Check sheet for the modelled part. Datum: model origin and axes. Units: mm. Face numbers are marked on the shaded views. A direction names the side the tool comes from. Round coordinates to 2 decimals unless told otherwise and drop trailing zeros. Write each loop counter-clockwise with the first axis right and the second up, starting at its lowest first coordinate (ties: lowest second). Pieces come first, ordered by that corner, then holes.
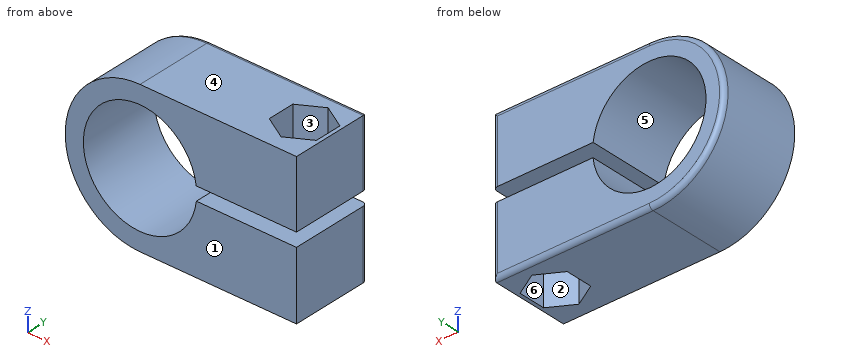
from build123d import *

# Parameters (mm, degrees)
BOSS_EXTRUDE1_DEPTH = 18
FILLET1_R           = 1
CUT_EXTRUDE1_START  = -10
CUT_EXTRUDE1_DEPTH  = 62.022054055


with BuildPart() as part:
    # Sketch1 → Boss-Extrude1 (new body)
    with BuildSketch(Plane(origin=(0, 0, 0), x_dir=(1, 0, 0), z_dir=(0, 1, 0))):
        with BuildLine():
            Line((0, -16.5), (34.5, -16.5))
            Line((34.5, -16.5), (34.5, -1.605540399))
            Line((34.5, -1.605540399), (12.396460786, -1.605540399))
            ThreePointArc((12.396460786, -1.605540399), (-12.499547931, 0.106308653), (12.421975786, 1.394459601))
            Line((12.421975786, 1.394459601), (34.5, 1.394459601))
            Line((34.5, 1.394459601), (34.5, 16.5))
            Line((34.5, 16.5), (0, 16.5))
            ThreePointArc((0, 16.5), (-16.5, 0), (0, -16.5))
        make_face()
    extrude(amount=BOSS_EXTRUDE1_DEPTH)

    # Fillet1
    fillet1_edges = [part.edges().sort_by_distance(p)[0] for p in [
        (17.25, 18, -16.5),
        (-16.5, 18, 0),
        (17.25, 18, 16.5),
        (34.5, 18, 9.0527702),
        (34.5, 18, -8.9472298),
    ]]
    fillet(fillet1_edges, radius=FILLET1_R)

    # Sketch2 → Cut-Extrude1 (cut)
    with BuildSketch(Plane.XY.offset(16.5).offset(CUT_EXTRUDE1_START)):
        Polygon((28.5, 15), (23.303847577, 12), (23.303847577, 6), (28.5, 3), (33.696152423, 6), (33.696152423, 12), align=None)
    cut_extrude1 = extrude(amount=CUT_EXTRUDE1_DEPTH, mode=Mode.SUBTRACT)

    # Mirror1: Cut-Extrude1 across plane
    add(cut_extrude1.mirror(Plane.XY), mode=Mode.SUBTRACT)


solid = part.part
1. Release check for a two-part mould opening along Z. For the marked faces 4, 5 and 6 record: released by +Z, released by -Z, zero draft, split by the parting line, or undercut.
2. Scan lines: line 1 along Z through (x, y) = (16, 16.5); line 2 along Z through (x, y) = (0, 13.5); line 3 along X through (y, z) = (5, 11.5). Record each from-to range of solid material in increasing order.
3. Set-up check for the marked faces 1, 2 and 3: record each of +Z, -Z, +X, -X, +Y, -Y from which the full face is reachable in a straight line by a thin tool's end or side.
4. Go/stop test with flat-tipped pins: pin 1 (5 mm diameter, centred on y = 9, z = 11, fed in from -X); pin 2 (1 mm diameter, centred on x = 14, z = 6.5, fed in from -Y); pin 3 (3 mm diameter, centred on x = 29, y = 7.5, fed in from -Z). Record where each tip stops, or that it passes through.
5. Sectioned sample at D-D, the plane z = 11. Give the number of separate pieces and of enclosed holes in the cut face, plus the area to 3 significant figures.
6. Sectioned sample at A-A, the plane x = 18. Enter the section's corners in (y, z).
7. Sectioned sample at B-B, the plane y = 7.75. Enter the section's corners in (x, z).
8. Sectioned sample at C-C, the plane x = 26. Enter the section's corners in (y, z), plus the area to 3 significant figures.
Computed values:
1. face 4: released by +Z
1. face 5: undercut
1. face 6: zero draft
2. line 1: z = -16.5 to -1.39, 1.61 to 16.5
2. line 2: z = -16.5 to -12.5, 12.5 to 16.5
2. line 3: x = -11.83 to -4.9, 4.9 to 25.04, 31.96 to 34.5
3. face 1: +Z, -Z, +X, -X, -Y
3. face 2: -Z
3. face 3: +Z
4. pin 1: stops at x = -14.14
4. pin 2: stops at y = 0
4. pin 3: stops at z = -6.5
5. separate pieces: 2
5. enclosed holes: 1
5. area: 535 mm2
6. outline: (0, -16.5) - (17, -16.5) arc R1 ccw to (18, -15.5) - (18, -1.39) - (0, -1.39) - close; (0, 1.61) - (18, 1.61) - (18, 15.5) arc R1 ccw to (17, 16.5) - (0, 16.5) - close
7. outline: (0, -16.5) - (23.3, -16.5) - (23.3, -6.5) - (33.7, -6.5) - (33.7, -16.5) - (34.5, -16.5) - (34.5, -1.39) - (12.42, -1.39) arc R12.5 cw (long way) to (12.4, 1.61) - (34.5, 1.61) - (34.5, 16.5) - (33.7, 16.5) - (33.7, 6.5) - (23.3, 6.5) - (23.3, 16.5) - (0, 16.5) arc R16.5 ccw to start
8. outline: (0, -16.5) - (4.44, -16.5) - (4.44, -6.5) - (13.56, -6.5) - (13.56, -16.5) - (17, -16.5) arc R1 ccw to (18, -15.5) - (18, -1.39) - (0, -1.39) - close; (0, 1.61) - (18, 1.61) - (18, 15.5) arc R1 ccw to (17, 16.5) - (13.56, 16.5) - (13.56, 6.5) - (4.44, 6.5) - (4.44, 16.5) - (0, 16.5) - close
8. area: 357 mm2
